Input: part model. Units: mm. Frame: model coordinates. Face numbers are marked on the shaded views. Coordinates: 2 decimals unless noted, no trailing zeros. Loops run counter-clockwise (first coordinate to the right, second up) from the corner with the lowest first, then second, coordinate; pieces in that order, holes last. Notation, with made-up numbers: (29, -1.5) -> (74, -1.5) arc R34 cw to (74, 30.5) -> close; hole circle Ø7 at (89, -17.5). An arc over 180 degrees is marked (long way). Answer as a JSON object with one key per item and string values.
from build123d import *

# Parameters (mm, degrees)
SKETCH1_W                                     = 12.6
SKETCH1_H                                     = 2
FOUR_THROUGH_HOLES_BOTH_DIRECTIONS_DEPTH      = 18.93097878
FOUR_THROUGH_HOLES_BOTH_DIRECTIONS_DEPTH_BACK = 18.93097878
SMA_D6_5_HOSES_D7_2_VENT_D2_R                 = 3.6
SMA_D6_5_HOSES_D7_2_VENT_D2_R_2               = 1


with BuildPart() as part:
    # Sketch1 → Revolve1 (revolve)
    with BuildSketch(Plane.XY, mode=Mode.PRIVATE) as revolve1_sk:
        with Locations((6.3, 1)):
            Rectangle(SKETCH1_W, SKETCH1_H)
    revolve(revolve1_sk.sketch.rotate(Axis((0, -200, 0), (0, 1, 0)), 90), axis=Axis((0, -200, 0), (0, 1, 0)))

    # SMA D6.5 - hoses D7.2 - vent D2 → Four through holes - both directions (cut, two sides: drawn at the far end of the back side and taken through both)
    with BuildSketch(Plane(origin=(0, 0, 0), x_dir=(1, 0, 0), z_dir=(0, 1, 0)).offset(-FOUR_THROUGH_HOLES_BOTH_DIRECTIONS_DEPTH_BACK)):
        with Locations(Location((-5.4, 3.6, 0), (0, 0, 270))):
            Circle(SMA_D6_5_HOSES_D7_2_VENT_D2_R)
        with Locations(Location((5.4, 3.6, 0), (0, 0, 270))):
            Circle(SMA_D6_5_HOSES_D7_2_VENT_D2_R)
        with Locations(Location((0, 9, 0), (0, 0, 270))):
            Circle(SMA_D6_5_HOSES_D7_2_VENT_D2_R_2)
        with BuildLine():
            Line((-1.732050808, -1.75), (1.732050808, -1.75))
            ThreePointArc((1.732050808, -1.75), (0, -7.75), (-1.732050808, -1.75))
        make_face()
    extrude(amount=FOUR_THROUGH_HOLES_BOTH_DIRECTIONS_DEPTH + FOUR_THROUGH_HOLES_BOTH_DIRECTIONS_DEPTH_BACK, mode=Mode.SUBTRACT)


solid = part.part
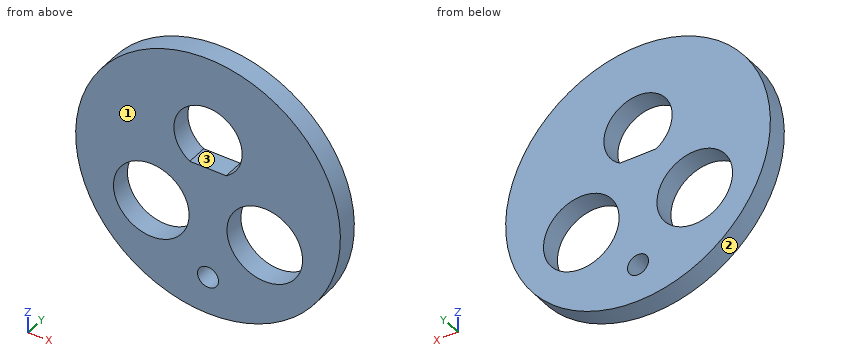
1. Section query B-B (z = 5.75). Return loops of the section in (x, y), plus the area to 3 significant figures.
Reply:
{"outline": "(-11.21, 0) -> (-3, 0) -> (-3, 2) -> (-11.21, 2) -> close; (3, 0) -> (11.21, 0) -> (11.21, 2) -> (3, 2) -> close", "area": "32.8 mm2"}
2. Section query C-C (x = -8.25). Return loops of the section in (y, z).
Reply:
{"outline": "(0, -9.52) -> (2, -9.52) -> (2, -5.8) -> (0, -5.8) -> close; (0, -1.4) -> (2, -1.4) -> (2, 9.52) -> (0, 9.52) -> close"}
3. Line query: line 1 along Z through (x, y) = (0.25, 0.35); line 2 along X through (y, z) = (0.1, -0.75); line 3 along X through (y, z) = (1.3, -2). Output: solid intervals per line, ascending.
Reply:
{"line 1": "z = -12.6 to -9.97, -8.03 to 1.75, 7.74 to 12.6", "line 2": "x = -12.58 to -7.6, -3.2 to 3.2, 7.6 to 12.58", "line 3": "x = -12.44 to -8.62, -2.18 to 2.18, 8.62 to 12.44"}
4. Pin query (flat end, axial travel): P1, Ø5, axis at x = 0, z = 4.5, coming from the -Y side. Return the tip coordinate at first contact, or that it passes through.
Reply:
{"P1": "passes through"}
5. Section query A-A (x = 0). Return loops of the section in (y, z).
Reply:
{"outline": "(0, -12.6) -> (2, -12.6) -> (2, -10) -> (0, -10) -> close; (0, -8) -> (2, -8) -> (2, 1.75) -> (0, 1.75) -> close; (0, 7.75) -> (2, 7.75) -> (2, 12.6) -> (0, 12.6) -> close"}
6. Section query D-D (y = 1.7). Return loops of the section in (x, z).
Reply:
{"outline": "circle Ø25.2 at (0, 0); hole circle Ø7.2 at (-5.4, -3.6); hole (-1.73, 1.75) -> (1.73, 1.75) arc R3.25 ccw (long way) to start; hole circle Ø2 at (0, -9); hole circle Ø7.2 at (5.4, -3.6)"}
7. Mould query, pull axis X, two halves, no side actions, for the marked faces 1, 2 and 3. Classes: pulls with the +X half, pulls with the -X half, needs draft (parallel to the pull), parting line crosses it, or undercut.
Reply:
{"face 1": "needs draft", "face 2": "parting line crosses it", "face 3": "undercut"}
